The drawing under review shows one solid part. Ordinate dimensions are in mm from its lowest x, y, z. A direction names the side the tool comes from. Coordinates: 2 decimals unless noted, no trailing zeros. Write each loop counter-clockwise with the first axis right and the second up, starting at its lowest first coordinate (ties: lowest second). Pieces come first, ordered by that corner, then holes. Notation, with made-up numbers: (76.25, -35.75) -> (133.25, -35.75) arc R26 cw to (133.25, -21.75) -> close; hole circle Ø10 at (18, 37). An arc over 180 degrees is marked (long way). Put each result on its own line as item: value. Start each with the question number.
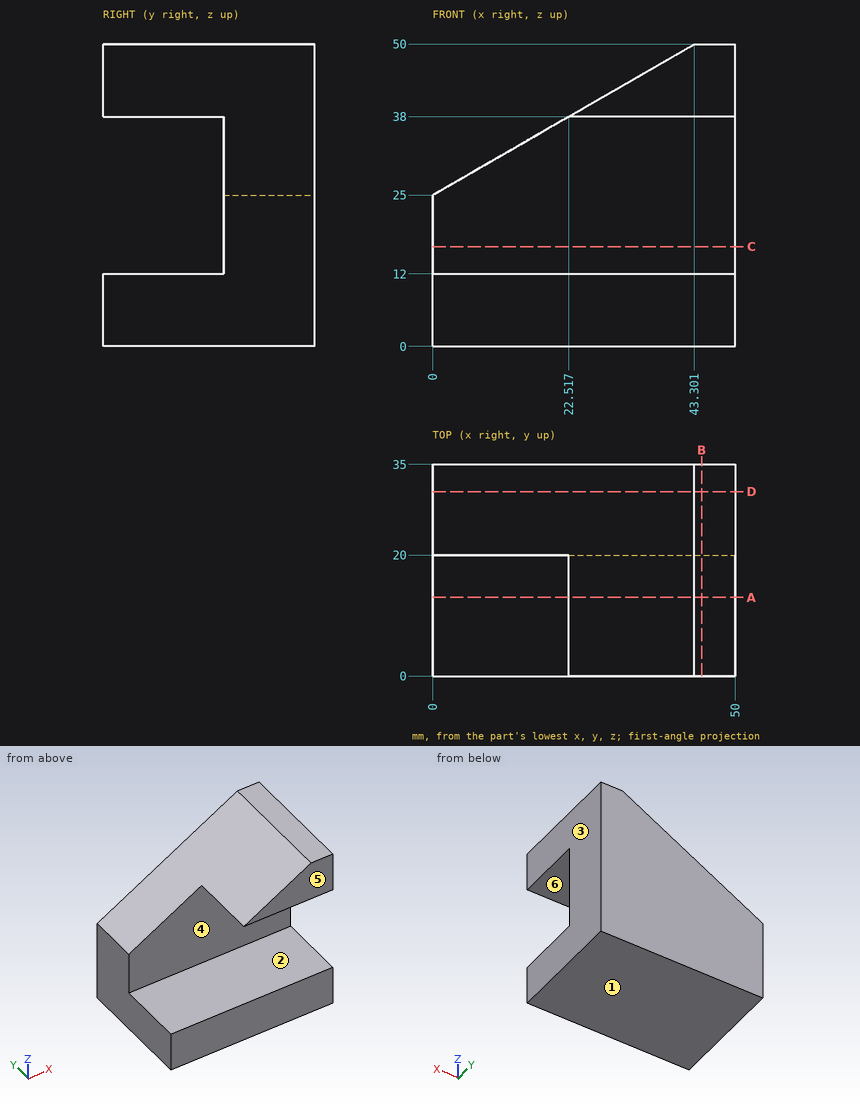
1. Tool access review of the marked faces 5 and 6: name each direction out of +Z, -Z, +X, -X, +Y, -Y from which nothing blocks a thin tool from reaching the whole face with its end or side.
2. Consider section B-B on x = 44.5. State the section outline as (y, z) points.
3. Consider section D-D on y = 30.5. State the section outline as (x, z) points.
4. Consider section A-A on y = 13. State the section outline as (x, z) points, then the cut area to 3 significant figures.
5. Wall thickness on line 1 (Z direction, x = 31.5, y = 13); line 2 (Y direction, x = 5.5, z = 22); line 3 (Z direction, x = 25.5, y = 12.5): over which ranges is each line inside the solid? List them lowest first. Write a range as from..to.
6. The part is to be moulded in two halves that separate along Z. For the marked faces 1, 2, 3 and 4, say which applies: released by +Z, released by -Z, zero draft, split by the parting line, or undercut.
7. Insertion check: P1, Ø8, axis at x = 23.5, z = 22, coming from the -Y side; P2, Ø2, axis at x = 9.5, y = 15, coming from the +Z side; P3, Ø10, axis at x = 20.5, y = 7.5, coming from the +Z side; P4, Ø6, axis at x = 8, z = 35, coming from the +Y side. Each pin has a flat end and moves straight along its axis. Give the tip position at first contact, or say it passes through.
8. Consider section C-C on z = 16.5. State the section outline as (x, y) points.
Output values:
1. face 5: +Z, -Z, +X, -X, -Y
1. face 6: +X, -X, -Y
2. outline: (0, 0) -> (35, 0) -> (35, 50) -> (0, 50) -> (0, 38) -> (20, 38) -> (20, 12) -> (0, 12) -> close
3. outline: (0, 0) -> (50, 0) -> (50, 50) -> (43.3, 50) -> (0, 25) -> close
4. outline: (0, 0) -> (50, 0) -> (50, 12) -> (0, 12) -> close; (22.52, 38) -> (50, 38) -> (50, 50) -> (43.3, 50) -> close
4. area: 805 mm^2
5. line 1: z = 0..12, 38..43.19
5. line 2: y = 20..35
5. line 3: z = 0..12, 38..39.72
6. face 1: released by -Z
6. face 2: undercut
6. face 3: zero draft
6. face 4: undercut
7. P1: stops at y = 20
7. P2: stops at z = 12
7. P3: stops at z = 39.72
7. P4: passes through
8. outline: (0, 20) -> (50, 20) -> (50, 35) -> (0, 35) -> close
